```python
from build123d import *

# Parameters (mm, degrees)
F0_W           = 180
F0_H           = 180
F1_DEPTH       = 70
F2_T           = -5
F3_W           = 170
F3_H           = 170
F4_DEPTH       = 10
F5_W           = 155
F5_H           = 155
F6_DEPTH       = 5
F7_W           = 145
F7_H           = 145
F8_DEPTH       = 25
F9_W           = 20
F9_H           = 20
F10_DEPTH      = 5
F11_W          = 236.9226813316
F11_H          = 264.4580230117
F11_W_2        = 180
F11_H_2        = 180
F12_DEPTH      = 25
F13_W          = 243.9718917012
F13_H          = 319.6009546518
F13_W_2        = 180
F13_H_2        = 180
F14_DEPTH      = 55
F14_DEPTH_BACK = 25
F15_W          = 192
F15_H          = 192
F15_W_2        = 180
F15_H_2        = 180
F16_DEPTH      = 10
F16_DEPTH_BACK = 10
F17_DEPTH      = 5
F18_W          = 186
F18_H          = 186
F18_W_2        = 180
F18_H_2        = 180
F19_DEPTH      = 10


with BuildPart() as f1:
    # F0 (on Top) → F1 (new body)
    with BuildSketch(Plane.XY):
        Rectangle(F0_W, F0_H)
    extrude(amount=F1_DEPTH)

    # F2
    f2_openings = [f1.faces().sort_by_distance(p)[0] for p in [
        (0, 0, 70),
    ]]
    offset(amount=F2_T, openings=f2_openings)

    # F3 (on face) → F4 (join)
    with BuildSketch(Plane.XY.offset(70)):
        Rectangle(F3_W, F3_H)
    extrude(amount=-F4_DEPTH)

    # F5 (on face) → F6 (cut)
    with BuildSketch(Plane.XY.offset(70)):
        Rectangle(F5_W, F5_H)
    extrude(amount=-F6_DEPTH, mode=Mode.SUBTRACT)

    # F7 (on face) → F8 (cut)
    with BuildSketch(Plane.XY.offset(65)):
        Rectangle(F7_W, F7_H)
    extrude(amount=-F8_DEPTH, mode=Mode.SUBTRACT)

    # F9 (on face) → F10 (join)
    with BuildSketch(Plane.XY.offset(65)):
        with Locations((-62.5, 62.5)):
            Rectangle(F9_W, F9_H)
        with Locations((62.5, 62.5)):
            Rectangle(F9_W, F9_H)
        with Locations((62.5, -62.5)):
            Rectangle(F9_W, F9_H)
        with Locations((-62.5, -62.5)):
            Rectangle(F9_W, F9_H)
    extrude(amount=-F10_DEPTH)

    # F11 (on face) → F12 (cut)
    with BuildSketch(Plane(origin=(0, 0, 0), x_dir=(1, 0, 0), z_dir=(0, 0, -1))):
        with Locations((12.1972411871, 16.292501241)):
            Rectangle(F11_W, F11_H)
        Rectangle(F11_W_2, F11_H_2, mode=Mode.SUBTRACT)
    extrude(amount=-F12_DEPTH, mode=Mode.SUBTRACT)

    # F13 (on face) → F14 (cut, two sides)
    with BuildSketch(Plane(origin=(0, 0, 0), x_dir=(1, 0, 0), z_dir=(0, 0, -1))) as f14_sk:
        with Locations((-22.6087830961, -21.1053714156)):
            Rectangle(F13_W, F13_H)
        Rectangle(F13_W_2, F13_H_2, mode=Mode.SUBTRACT)
        Rectangle(F13_W_2, F13_H_2)
    extrude(amount=-F14_DEPTH, mode=Mode.SUBTRACT)
    extrude(f14_sk.sketch, amount=F14_DEPTH_BACK, mode=Mode.SUBTRACT)

    # F15 (on face) → F16 (join, two sides)
    with BuildSketch(Plane(origin=(0, 0, 60), x_dir=(1, 0, 0), z_dir=(0, 0, -1))) as f16_sk:
        Rectangle(F15_W, F15_H)
        Rectangle(F15_W_2, F15_H_2, mode=Mode.SUBTRACT)
    extrude(amount=F16_DEPTH)
    extrude(f16_sk.sketch, amount=-F16_DEPTH_BACK)

    # F17 (cut, through all): a face of the model
    f17_faces = [f1.faces().sort_by_distance(p)[0] for p in [
        (87.4544155877, 0, 55),
    ]]
    extrude(f17_faces, amount=-F17_DEPTH, mode=Mode.SUBTRACT)

    # F18 (on face) → F19 (cut, through all)
    with BuildSketch(Plane(origin=(0, 0, 50), x_dir=(1, 0, 0), z_dir=(0, 0, -1))):
        Rectangle(F18_W, F18_H)
        Rectangle(F18_W_2, F18_H_2, mode=Mode.SUBTRACT)
        Rectangle(F18_W_2, F18_H_2)
    extrude(amount=-F19_DEPTH, mode=Mode.SUBTRACT)


solid = f1.part
```
Geometry check sheet. Reference: the model listing, model coordinates, mm. A direction names the side the tool comes from. Round coordinates to 2 decimals unless told otherwise and drop trailing zeros. Loops run counter-clockwise (first coordinate to the right, second up) from the corner with the lowest first, then second, coordinate; pieces in that order, holes last. Notation, with made-up numbers: (-22, 46.5) - (3, 46.5) arc R15 cw to (3, 66.5) - close; hole circle Ø11 at (27, 82). An arc over 180 degrees is marked (long way). Use a Markdown table: item, result.
Q1. Access from +Z, -Z, +X, -X, +Y, -Y to the whole of each face (thin tool, end or side, straight path). Record for faces 1 (the flat face through (-1, 72.5, 63)), 2 (the flat face through (77.5, -1, 68)), 3 (the flat face through (93, 1, 55)), 4 (the flat face through (84, -1, 70)), 5 (the flat face through (-1, 96, 60)).
Solutions:
| item | result |
|---|---|
| face 1 | +Z, -Z |
| face 2 | +Z |
| face 3 | -Z |
| face 4 | +Z, +X, -X, +Y, -Y |
| face 5 | +Z, -Z, +X, -X, +Y |
Q2. Draft check along X on faces 6 (the flat face through (96, 1, 60)), 7 (the flat face through (-84, -1, 60)), 8 (the flat face through (-63, 52.5, 63)), 9 (the flat face through (-96, 1, 60)). Enter one of: released by +X, released by -X, zero draft, split by the parting line, or undercut.
Solutions:
| item | result |
|---|---|
| face 6 | released by +X |
| face 7 | undercut |
| face 8 | undercut |
| face 9 | released by -X |
Q3. Material ranges on line 1 (X direction, y = 73.5, z = 68); line 2 (X direction, y = -25.5, z = 59), recorded low to high.
Solutions:
| item | result |
|---|---|
| line 1 | x = -96 to -77.5, 77.5 to 96 |
| line 2 | x = -96 to -93, 93 to 96 |
Q4. Cross-section at D-D on x = 82. Record the cut outline in (y, z), plus the area to 3 significant figures.
Solutions:
| item | result |
|---|---|
| outline | (-96, 50) - (-93, 50) - (-93, 60) - (93, 60) - (93, 50) - (96, 50) - (96, 70) - (-96, 70) - close |
| area | 1,980 mm2 |
Q5. Cross-section at C-C on z = 62.5. Record the cut outline in (x, y), plus the area to 3 significant figures.
Solutions:
| item | result |
|---|---|
| outline | (-96, -96) - (96, -96) - (96, 96) - (-96, 96) - close; hole (-72.5, -52.5) - (-52.5, -52.5) - (-52.5, -72.5) - (52.5, -72.5) - (52.5, -52.5) - (72.5, -52.5) - (72.5, 52.5) - (52.5, 52.5) - (52.5, 72.5) - (-52.5, 72.5) - (-52.5, 52.5) - (-72.5, 52.5) - close |
| area | 17,400 mm2 |
Q6. Go/stop test with a flat-tipped pin: P1, Ø4, axis at x = -68.5, y = -54, coming from the +Z side. Record where the tip stops, or that it passes through.
Solutions:
| item | result |
|---|---|
| P1 | stops at z = 65 |
Q7. Cross-section at A-A on y = -4.5. Record the cut outline in (x, z).
Solutions:
| item | result |
|---|---|
| outline | (-96, 50) - (-93, 50) - (-93, 60) - (-72.5, 60) - (-72.5, 65) - (-77.5, 65) - (-77.5, 70) - (-96, 70) - close; (72.5, 60) - (93, 60) - (93, 50) - (96, 50) - (96, 70) - (77.5, 70) - (77.5, 65) - (72.5, 65) - close |
